from build123d import *

# Parameters (mm, degrees)
SKETCH1_W               = 378
SKETCH1_H               = 16
BOSS_EXTRUDE1_DEPTH     = 6
CUT_EXTRUDE1_DEPTH      = 381.976768496
CUT_EXTRUDE1_DEPTH_BACK = 374
SKETCH3_W               = 4.3
SKETCH3_H               = 12.3
BOSS_EXTRUDE2_DEPTH     = 374
BOSS_EXTRUDE3_DEPTH     = 374
SKETCH6_W               = 4
SKETCH6_H               = 8.5
CUT_EXTRUDE2_DEPTH      = 378.00835287
FILLET2_R               = 3
SKETCH13_W              = 10
SKETCH13_H              = 15
BOSS_EXTRUDE5_DEPTH     = 4
FILLET9_R               = 3
FILLET10_R              = 4
SKETCH14_R              = 1.7
CUT_EXTRUDE5_DEPTH      = 4
FILLET11_R              = 4
FILLET12_R              = 4
LPATTERN3_COUNT         = 3
LPATTERN3_PITCH         = 172.5
LPATTERN4_COUNT         = 3
LPATTERN4_PITCH         = 172.5
FILLET13_R              = 4
FILLET14_R              = 4
FILLET15_R              = 3
FILLET16_R              = 4
FILLET17_R              = 4
FILLET18_R              = 4
FILLET19_R              = 4
FILLET20_R              = 2
FILLET21_R              = 2
FILLET22_R              = 2
FILLET23_R              = 3
SKETCH15_R              = 1
CUT_EXTRUDE6_DEPTH      = 0.5
FILLET24_R              = 0.5


# Some blends are built 0.0001 mm under size
with BuildPart() as part:
    # Sketch1 → Boss-Extrude1 (new body)
    with BuildSketch(Plane.XY):
        with Locations((31.46991404, 39.151862464)):
            Rectangle(SKETCH1_W, SKETCH1_H)
    extrude(amount=BOSS_EXTRUDE1_DEPTH)

    # Sketch3 → Cut-Extrude1 (cut, two sides: drawn at the far end of the back side and taken through both)
    with BuildSketch(Plane(origin=(220.46991404, 0, 0), x_dir=(0, 0, -1), z_dir=(1, 0, 0)).offset(-CUT_EXTRUDE1_DEPTH_BACK)):
        with Locations((-3.85, 39.151862464)):
            Rectangle(SKETCH3_W, SKETCH3_H)
    extrude(amount=CUT_EXTRUDE1_DEPTH + CUT_EXTRUDE1_DEPTH_BACK, mode=Mode.SUBTRACT)

    # Sketch4 → Boss-Extrude2 (add)
    with BuildSketch(Plane(origin=(220.46991404, 0, 0), x_dir=(0, 0, -1), z_dir=(1, 0, 0))):
        Polygon((-6, 33.001862464), (-6, 34.001862464), (-5, 33.001862464), align=None)
    extrude(amount=-BOSS_EXTRUDE2_DEPTH)

    # Sketch5 → Boss-Extrude3 (add)
    with BuildSketch(Plane(origin=(220.46991404, 0, 0), x_dir=(0, 0, -1), z_dir=(1, 0, 0))):
        Polygon((-6, 45.301862464), (-6, 44.301862464), (-5, 45.301862464), align=None)
    extrude(amount=-BOSS_EXTRUDE3_DEPTH)

    # Sketch6 → Cut-Extrude2 (cut, through all)
    with BuildSketch(Plane(origin=(-153.53008596, 0, 0), x_dir=(0, 0, -1), z_dir=(1, 0, 0))):
        with Locations((-4, 39.151862464)):
            Rectangle(SKETCH6_W, SKETCH6_H)
    extrude(amount=-CUT_EXTRUDE2_DEPTH, mode=Mode.SUBTRACT)

    # Fillet2
    # the kernel refuses this fillet: 3 mm, written as the material it takes off along each edge
    with BuildSketch(Plane(origin=(-157.53008596, 23.651862464, 0), x_dir=(0, 0, 1), z_dir=(0, 1, 0))) as fillet2_piece_1:
        with BuildLine():
            CenterArc((FILLET2_R, FILLET2_R), FILLET2_R, 180, 90)
            Line((0, FILLET2_R), (0, 0))
            Line((0, 0), (FILLET2_R, 0))
        make_face()
    extrude(amount=31, mode=Mode.SUBTRACT)

    # Sketch13 → Boss-Extrude5 (add)
    with BuildSketch(Plane(origin=(0, 47.151862464, 0), x_dir=(1, 0, 0), z_dir=(0, 1, 0))):
        with Locations((-142.53008596, -7.5)):
            Rectangle(SKETCH13_W, SKETCH13_H)
    boss_extrude5 = extrude(amount=BOSS_EXTRUDE5_DEPTH)

    # Fillet9
    fillet9_edges = [part.edges().sort_by_distance(p)[0] for p in [
        (32.96991404, 31.151862464, 0),
        (-156.651406303, 31.151862464, 0.878679656),
        (-157.53008596, 31.151862464, 4.5),
    ]]
    fillet(fillet9_edges, radius=FILLET9_R)

    # Fillet10
    fillet10_edges = [part.edges().sort_by_distance(p)[0] for p in [
        (-142.53008596, 51.151862464, 0),
    ]]
    fillet(fillet10_edges, radius=FILLET10_R)

    # Sketch14 → Cut-Extrude5 (cut)
    with BuildSketch(Plane.XZ.offset(-47.151862464)):
        with Locations(Location((-142.53008596, 10, 0), (0, 0, 270))):
            Circle(SKETCH14_R)
    cut_extrude5 = extrude(amount=-CUT_EXTRUDE5_DEPTH, mode=Mode.SUBTRACT)

    # Fillet11
    fillet11_edges = [part.edges().sort_by_distance(p)[0] for p in [
        (-137.53008596, 49.151862464, 15),
    ]]
    fillet(fillet11_edges, radius=FILLET11_R)

    # Fillet12
    fillet12_edges = [part.edges().sort_by_distance(p)[0] for p in [
        (-147.53008596, 49.151862464, 15),
    ]]
    fillet(fillet12_edges, radius=FILLET12_R)

    # LPattern3: Boss-Extrude5 ×3
    with Locations(*[(i * LPATTERN3_PITCH, 0, 0) for i in range(1, LPATTERN3_COUNT)]):
        add(boss_extrude5)

    # LPattern4: Cut-Extrude5 ×3
    with Locations(*[(i * LPATTERN4_PITCH, 0, 0) for i in range(1, LPATTERN4_COUNT)]):
        add(cut_extrude5, mode=Mode.SUBTRACT)

    # Fillet13
    fillet13_edges = [part.edges().sort_by_distance(p)[0] for p in [
        (29.96991404, 51.151862464, 0),
    ]]
    fillet(fillet13_edges, radius=FILLET13_R)

    # Fillet14
    fillet14_edges = [part.edges().sort_by_distance(p)[0] for p in [
        (202.46991404, 51.151862464, 0),
    ]]
    fillet(fillet14_edges, radius=FILLET14_R)

    # Fillet15
    # the kernel refuses this fillet: 3 mm, written as the material it takes off along each edge
    with BuildSketch(Plane(origin=(34.96991404, 47.151862464, 0), x_dir=(0, -1, 0), z_dir=(1, 0, 0)), Plane(origin=(-137.53008596, 47.151862464, 0), x_dir=(0, -1, 0), z_dir=(1, 0, 0))) as fillet15_piece_1:
        with BuildLine():
            CenterArc((FILLET15_R, -FILLET15_R), FILLET15_R, 90, 90)
            Line((0, -FILLET15_R), (0, 0))
            Line((0, 0), (FILLET15_R, 0))
        make_face()
    extrude(amount=162.5, mode=Mode.SUBTRACT)
    with BuildSketch(Plane(origin=(207.46991404, 47.151862464, 0), x_dir=(0, -1, 0), z_dir=(1, 0, 0))) as fillet15_piece_2:
        with BuildLine():
            CenterArc((FILLET15_R, -FILLET15_R), FILLET15_R, 90, 90)
            Line((0, -FILLET15_R), (0, 0))
            Line((0, 0), (FILLET15_R, 0))
        make_face()
    extrude(amount=20.5, mode=Mode.SUBTRACT)
    with BuildSketch(Plane(origin=(-157.53008596, 47.151862464, 3), x_dir=(1, 0, 0), z_dir=(0, 0, 1))) as fillet15_piece_3:
        with BuildLine():
            CenterArc((FILLET15_R, -FILLET15_R), FILLET15_R, 90, 90)
            Line((0, -FILLET15_R), (0, 0))
            Line((0, 0), (FILLET15_R, 0))
        make_face()
    extrude(amount=10.5, mode=Mode.SUBTRACT)
    with BuildSketch(Plane(origin=(-154.53008596, 47.151862464, 3), x_dir=(-1, 0, 0), z_dir=(0, 0, 1))) as fillet15_piece_4:
        with BuildLine():
            CenterArc((3 - FILLET15_R, FILLET15_R), FILLET15_R, 270, 90)
            Line((3 - FILLET15_R, 0), (3, 0))
            Line((3, 0), (3, FILLET15_R))
        make_face()
    revolve(axis=Axis((-154.53008596, 47.151862464, 3), (0, -1, 0)), revolution_arc=90, mode=Mode.SUBTRACT)
    with BuildSketch(Plane(origin=(-154.53008596, 47.151862464, 0), x_dir=(0, -1, 0), z_dir=(1, 0, 0))) as fillet15_piece_5:
        with BuildLine():
            CenterArc((FILLET15_R, -FILLET15_R), FILLET15_R, 90, 90)
            Line((0, -FILLET15_R), (0, 0))
            Line((0, 0), (FILLET15_R, 0))
        make_face()
    extrude(amount=7, mode=Mode.SUBTRACT)

    # Fillet16
    fillet16_edges = [part.edges().sort_by_distance(p)[0] for p in [
        (24.96991404, 49.151862464, 15),
    ]]
    fillet(fillet16_edges, radius=FILLET16_R)

    # Fillet17
    fillet17_edges = [part.edges().sort_by_distance(p)[0] for p in [
        (34.96991404, 49.151862464, 15),
    ]]
    fillet(fillet17_edges, radius=FILLET17_R)

    # Fillet18
    fillet18_edges = [part.edges().sort_by_distance(p)[0] for p in [
        (207.46991404, 49.151862464, 15),
    ]]
    fillet(fillet18_edges, radius=FILLET18_R)

    # Fillet19
    fillet19_edges = [part.edges().sort_by_distance(p)[0] for p in [
        (197.46991404, 49.151862464, 15),
    ]]
    fillet(fillet19_edges, radius=FILLET19_R)

    # Fillet20
    fillet20_edges = [part.edges().sort_by_distance(p)[0] for p in [
        (202.46991404, 47.151862464, 6),
    ]]
    fillet(fillet20_edges, radius=FILLET20_R)

    # Fillet21
    fillet21_edges = [part.edges().sort_by_distance(p)[0] for p in [
        (29.96991404, 47.151862464, 6),
    ]]
    fillet(fillet21_edges, radius=FILLET21_R)

    # Fillet22
    fillet22_edges = [part.edges().sort_by_distance(p)[0] for p in [
        (-142.53008596, 47.151862464, 6),
    ]]
    fillet(fillet22_edges, radius=FILLET22_R)

    # Fillet23
    # the kernel refuses this fillet: 3 mm, written as the material it takes off along each edge
    with BuildSketch(Plane(origin=(220.46991404, 31.151862464, 3), x_dir=(0, 1, 0), z_dir=(0, 0, 1))) as fillet23_piece_1:
        with BuildLine():
            CenterArc((FILLET23_R, FILLET23_R), FILLET23_R, 180, 90)
            Line((0, FILLET23_R), (0, 0))
            Line((0, 0), (FILLET23_R, 0))
        make_face()
    extrude(amount=10.5, mode=Mode.SUBTRACT)
    with BuildSketch(Plane(origin=(220.46991404, 34.151862464, 3), x_dir=(0, 0, -1), z_dir=(0, 1, 0))) as fillet23_piece_2:
        with BuildLine():
            CenterArc((3 - FILLET23_R, FILLET23_R), FILLET23_R, 270, 90)
            Line((3, FILLET23_R), (3, 0))
            Line((3, 0), (3 - FILLET23_R, 0))
        make_face()
    revolve(axis=Axis((220.46991404, 34.151862464, 3), (-1, 0, 0)), revolution_arc=90, mode=Mode.SUBTRACT)
    with BuildSketch(Plane(origin=(220.46991404, 47.151862464, 3), x_dir=(0, -1, 0), z_dir=(0, 0, 1))) as fillet23_piece_3:
        with BuildLine():
            CenterArc((FILLET23_R, -FILLET23_R), FILLET23_R, 90, 90)
            Line((0, -FILLET23_R), (0, 0))
            Line((0, 0), (FILLET23_R, 0))
        make_face()
    extrude(amount=10.5, mode=Mode.SUBTRACT)
    with BuildSketch(Plane(origin=(220.46991404, 44.151862464, 3), x_dir=(0, 1, 0), z_dir=(0, 0, 1))) as fillet23_piece_4:
        with BuildLine():
            CenterArc((3 - FILLET23_R, FILLET23_R), FILLET23_R, 270, 90)
            Line((3, FILLET23_R), (3, 0))
            Line((3, 0), (3 - FILLET23_R, 0))
        make_face()
    revolve(axis=Axis((220.46991404, 44.151862464, 3), (-1, 0, 0)), revolution_arc=90, mode=Mode.SUBTRACT)
    with BuildSketch(Plane(origin=(220.46991404, 44.151862464, 0), x_dir=(0, 0, 1), z_dir=(0, -1, 0))) as fillet23_piece_5:
        with BuildLine():
            CenterArc((FILLET23_R, FILLET23_R), FILLET23_R, 180, 90)
            Line((0, FILLET23_R), (0, 0))
            Line((0, 0), (FILLET23_R, 0))
        make_face()
    extrude(amount=10, mode=Mode.SUBTRACT)

    # Sketch15 → Cut-Extrude6 (cut)
    with BuildSketch(Plane.XY.offset(1.7)):
        with Locations((218.173615207, 39.151862464)):
            Circle(SKETCH15_R)
    extrude(amount=-CUT_EXTRUDE6_DEPTH, mode=Mode.SUBTRACT)

    # Fillet24
    fillet24_edges = [part.edges().sort_by_distance(p)[0] for p in [
        (217.173615207, 39.151862464, 1.7),
    ]]
    fillet(fillet24_edges, radius=FILLET24_R - 0.0001)  # a hair under: the kernel refuses the full size


solid = part.part
Here's how the part is built. I have some questions about the finished solid (model axes, mm). A direction names the side the tool comes from. Give positions to 0.01 mm unless a question says otherwise; leave off trailing zeros. Order: outer loops, then holes, each group sorted by start corner. A loop starts at its lowest first (then second) coordinate and runs counter-clockwise, first axis right, second up. Notation, with made-up numbers: (7, 23) -> (16, 23) arc R16 ccw to (16, 40) -> close; hole circle Ø7 at (34, 33). An arc over 180 degrees is marked (long way). Use a Markdown table: item, result. Add a question column.
Item 1: If we mould it in two halves opening along X, with no side actions, what happens to faces 1 (the face through (29, 39, 0)), 2 (the face through (197.47, 49, 5)), 3 (the face through (207.47, 49, 5))? For each: pulls with the +X half, pulls with the -X half, needs draft (parallel to the pull), parting line crosses it, or undercut.
Item 2: Imagine slicing it at A-A on x = -20.5. Please give me the cut outline in (y, z).
Item 3: I need wall thicknesses on line 1 (X direction, y = 48.5, z = 4); line 2 (X direction, y = 48.2, z = 10); line 3 (Y direction, x = 32.5, z = 3.25). Which ranges of each line are inside material? Lowest first, please.
Item 4: For faces 4 (the face through (202, 47.152, 12)), 5 (the face through (31, 39, 1.7)), 6 (the face through (202, 51.152, 8)), which set-ups out of +Z, -Z, +X, -X, +Y, -Y let a thin tool reach every point of the face, with its end or its side?
Item 5: Will these pins go through, and if not, where does the flat tip stop? pin 1 (2 mm diameter, centred on y = 43, z = 6, fed in from +X); pin 2 (0.6 mm diameter, centred on x = 218, y = 39, fed in from +Z); pin 3 (1.9 mm diameter, centred on x = 113, y = 32.5, fed in from +Z).
Data:
| question | item | result |
|---|---|---|
| 1 | face 1 | needs draft |
| 1 | face 2 | undercut |
| 1 | face 3 | pulls with the +X half |
| 2 | outline | (31.15, 3) arc R3 ccw to (34.15, 0) -> (44.15, 0) arc R3 ccw to (47.15, 3) -> (47.15, 6) -> (44.3, 6) -> (45.3, 5) -> (45.3, 1.7) -> (33, 1.7) -> (33, 5) -> (34, 6) -> (31.15, 6) -> close |
| 3 | line 1 | x = -147.53 to -137.53, 24.97 to 34.97, 197.47 to 207.47 |
| 3 | line 2 | x = -147.53 to -144.23, -140.83 to -137.53, 24.97 to 28.27, 31.67 to 34.97, 197.47 to 200.77, 204.17 to 207.47 |
| 3 | line 3 | y = 31.15 to 33, 45.3 to 51.08 |
| 4 | face 4 | +Z, +X, -X, -Y |
| 4 | face 5 | +X |
| 4 | face 6 | +Z, -Z, +X, -X, +Y |
| 5 | pin 1 | stops at x = -153.53 |
| 5 | pin 2 | stops at z = 1.2 |
| 5 | pin 3 | stops at z = 6 |
